Here's how the part is built. I have some questions about the finished solid (model axes, mm). Give positions to 0.01 mm unless a question says otherwise; leave off trailing zeros. Loops run counter-clockwise (first coordinate to the right, second up) from the corner with the lowest first, then second, coordinate; pieces in that order, holes last. Notation, with made-up numbers: M -16,-21 L 23,-21 A16 ccw 23,-17 Z; hole C -33,-36.75 d5. An arc over 180 degrees is marked long. Answer as CSV lines item,"result". Start each with the question number.
Item 1: I want a section at C-C on x = 2. List the corners of the cut face in (y, z) for me.
Item 2: I want a section at A-A on y = -25.5. List the corners of the cut face in (x, z) for me, plus the area to 3 significant figures.
Item 3: I want a section at B-B on x = 32. List the corners of the cut face in (y, z) for me.
Item 4: Will these pins go through, and if not, where does the flat tip stop? P1, Ø17.5, axis at x = -23.16, y = -13.4, coming from the -Z side; P2, Ø0.9, axis at y = 30.5, z = 1, coming from the -X side; P3, Ø1, axis at y = 19.5, z = 2.5, coming from the +X side; P4, Ø0.9, axis at x = 10, z = 1, coming from the -Y side.
Item 5: If I drill on line 1 along X through (y, z) = (4.5, 1.5); line 2 along Y through (x, z) = (-6.5, 2.7); line 3 along X through (y, z) = (1, 2.1), over which ranges is the centre line in solid material (lowest first)? Write a range as from..to.
Item 6: I want a section at D-D on z = 0.85. List the corners of the cut face in (x, y) for me, plus the area to 3 significant figures.
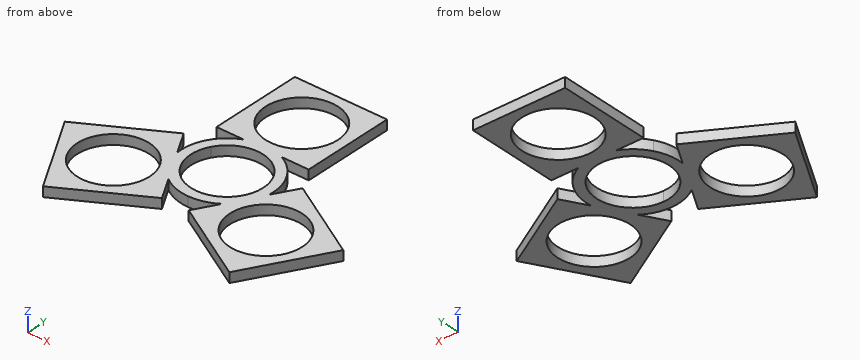
from build123d import *

# Parameters (mm, degrees)
F0_R     = 11
F1_DEPTH = 3


with BuildPart() as f1:
    # F0 (on Top) → F1 (new body)
    with BuildSketch(Plane.XY):
        with BuildLine():
            Line((-14.027199, 12.756373), (-5.768445, 12.756373))
            ThreePointArc((-5.768445, 12.756373), (-9.39798, 10.3768), (-12.124356, 7))
            ThreePointArc((-12.124356, 7), (-13.685562, 2.95049), (-13.931565, -1.382567))
            Line((-13.931565, -1.382567), (-18.033744, 5.722614))
            Line((-18.033744, 5.722614), (-42.282455, -8.277386))
            Line((-42.282455, -8.277386), (-28.282455, -32.526097))
            Line((-28.282455, -32.526097), (-4.033744, -18.526097))
            Line((-4.033744, -18.526097), (-8.163121, -11.373806))
            ThreePointArc((-8.163121, -11.373806), (-4.287582, -13.327289), (0, -14))
            ThreePointArc((0, -14), (4.287582, -13.327289), (8.163121, -11.373806))
            Line((8.163121, -11.373806), (4.060942, -18.478987))
            Line((4.060942, -18.478987), (28.309654, -32.478987))
            Line((28.309654, -32.478987), (42.309654, -8.230276))
            Line((42.309654, -8.230276), (18.060942, 5.769724))
            Line((18.060942, 5.769724), (13.931565, -1.382567))
            ThreePointArc((13.931565, -1.382567), (13.685562, 2.95049), (12.124356, 7))
            ThreePointArc((12.124356, 7), (9.39798, 10.3768), (5.768445, 12.756373))
            Line((5.768445, 12.756373), (13.972801, 12.756373))
            Line((13.972801, 12.756373), (13.972801, 40.756373))
            Line((13.972801, 40.756373), (-14.027199, 40.756373))
            Line((-14.027199, 40.756373), (-14.027199, 12.756373))
        make_face()
        with Locations((-23.158099, -13.401741)):
            Circle(F0_R, mode=Mode.SUBTRACT)
        with BuildLine():
            ThreePointArc((-9.526279, 5.5), (0, 11), (9.526279, 5.5))
            ThreePointArc((9.526279, 5.5), (9.526279, -5.5), (0, -11))
            ThreePointArc((0, -11), (-9.526279, -5.5), (-9.526279, 5.5))
        make_face(mode=Mode.SUBTRACT)
        with Locations((23.185298, -13.354632)):
            Circle(F0_R, mode=Mode.SUBTRACT)
        with Locations((-0.027199, 26.756373)):
            Circle(F0_R, mode=Mode.SUBTRACT)
    extrude(amount=F1_DEPTH)


solid = f1.part
Result:
1,outline,"M -13.86,0 L -10.82,0 L -10.82,3 L -13.86,3 Z; M 10.82,0 L 15.94,0 L 15.94,3 L 10.82,3 Z; M 37.57,0 L 40.76,0 L 40.76,3 L 37.57,3 Z"
2,outline,"M -32.34,0 L -16.11,0 L -16.11,3 L -32.34,3 Z; M 16.22,0 L 32.34,0 L 32.34,3 L 16.22,3 Z"
2,area,"97.0 mm^2"
3,outline,"M -26.09,0 L -19.93,0 L -19.93,3 L -26.09,3 Z; M -6.77,0 L -2.28,0 L -2.28,3 L -6.77,3 Z"
4,P1,"through"
4,P2,"x = -14.03"
4,P3,"x = 13.97"
4,P4,"y = -22.17"
5,line 1,"-20.15..-17.33, -13.26..-10.04, 10.04..13.26, 17.33..20.26"
5,line 2,"-19.95..-14.25, -12.4..-8.87, 8.87..12.4, 12.76..17.86, 35.65..40.76"
5,line 3,"-26.21..-15.31, -13.96..-10.95, 10.95..13.96, 15.31..26.32"
6,outline,"M -42.28,-8.28 L -28.28,-32.53 L -4.03,-18.53 L -8.16,-11.37 A14 ccw 0,-14 A14 ccw 8.16,-11.37 L 4.06,-18.48 L 28.31,-32.48 L 42.31,-8.23 L 18.06,5.77 L 13.93,-1.38 A14 ccw 12.12,7 A14 ccw 5.77,12.76 L 13.97,12.76 L 13.97,40.76 L -14.03,40.76 L -14.03,12.76 L -5.77,12.76 A14 ccw -12.12,7 A14 ccw -13.93,-1.38 L -18.03,5.72 Z; hole C -23.16,-13.4 d22; hole C -0.03,26.76 d22; hole C 0,0 d22; hole C 23.19,-13.35 d22"
6,area,"1,420 mm^2"
